from build123d import *

# Parameters (mm, degrees)
SKETCH1_W             = 45
SKETCH1_H             = 33
EXTRUDE1_DEPTH        = 45
EXTRUDE3_DEPTH        = 53.948087784
M5_TAPPED_HOLE1_D     = 4.2
M5_TAPPED_HOLE1_DEPTH = 10
M5_TAPPED_HOLE1_TIP   = 1.2618073
CHAMFER1_SIZE         = 1


with BuildPart() as part:
    # Sketch1 → Extrude1 (new body)
    with BuildSketch(Plane.XY):
        Rectangle(SKETCH1_W, SKETCH1_H)
    extrude(amount=EXTRUDE1_DEPTH)

    # Sketch2 → Extrude3 (cut, through all)
    with BuildSketch(Plane.XY.offset(45)):
        with BuildLine():
            Line((4.983173546, -10.386071552), (0, -4.447356576))
            Line((0, -4.447356576), (-4.983173546, -10.386071552))
            ThreePointArc((-4.983173546, -10.386071552), (0, -12), (4.983173546, -10.386071552))
        make_face()
        with BuildLine():
            Line((-4.983173546, -10.386071552), (0, -4.447356576))
            Line((0, -4.447356576), (4.983173546, -10.386071552))
            ThreePointArc((4.983173546, -10.386071552), (7.569906708, -7.366071964), (8.5, -3.5))
            ThreePointArc((8.5, -3.5), (-3.866071964, 4.069906708), (-4.983173546, -10.386071552))
        make_face()
        Polygon((10.113368652, -16.5), (-10.113368652, -16.5), (-13.53955506, -20.583169961), (13.53955506, -20.583169961), align=None)
        with BuildLine():
            ThreePointArc((4.983173546, -10.386071552), (0, -12), (-4.983173546, -10.386071552))
            Line((-4.983173546, -10.386071552), (-10.113368652, -16.5))
            Line((-10.113368652, -16.5), (10.113368652, -16.5))
            Line((10.113368652, -16.5), (4.983173546, -10.386071552))
        make_face()
    extrude(amount=-EXTRUDE3_DEPTH, mode=Mode.SUBTRACT)

    # M5 Tapped Hole1
    with Locations(Plane(origin=(0, 16.5, 0), x_dir=(-1, 0, 0), z_dir=(0, 1, 0))):
        with Locations((16, 7.5), (-16, 7.5), (-16, 37.5), (16, 37.5)):
            Hole(M5_TAPPED_HOLE1_D / 2, depth=M5_TAPPED_HOLE1_DEPTH)
            with Locations((0, 0, -(M5_TAPPED_HOLE1_DEPTH + M5_TAPPED_HOLE1_TIP / 2))):  # 118° drill point
                Cone(0, M5_TAPPED_HOLE1_D / 2, M5_TAPPED_HOLE1_TIP, mode=Mode.SUBTRACT)

    # Chamfer1
    chamfer1_edges = [part.edges().sort_by_distance(p)[0] for p in [
        (-22.5, 0, 45),
        (-16.306684326, -16.5, 45),
        (16.306684326, -16.5, 0),
        (16.306684326, -16.5, 45),
        (0, 5, 45),
        (0, 5, 0),
        (22.5, 0, 45),
        (-16.306684326, -16.5, 0),
        (-22.5, 0, 0),
        (0, 16.5, 0),
        (22.5, 0, 0),
        (0, 16.5, 45),
        (22.5, -16.5, 22.5),
        (-22.5, -16.5, 22.5),
        (-22.5, 16.5, 22.5),
        (22.5, 16.5, 22.5),
    ]]
    chamfer(chamfer1_edges, length=CHAMFER1_SIZE)


solid = part.part
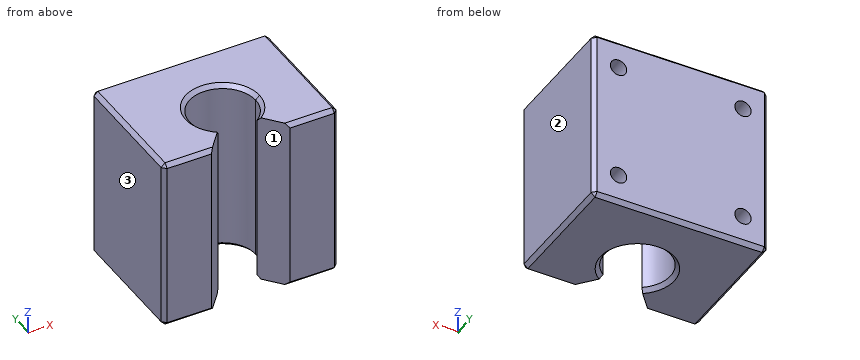
Model file for the job. Use its own axes, mm. Face numbers are marked on the shaded views. Give positions to 0.01 mm unless a question says otherwise; leave off trailing zeros. Order: outer loops, then holes, each group sorted by start corner. A loop starts at its lowest first (then second) coordinate and runs counter-clockwise, first axis right, second up. Notation, with made-up numbers: M 2.5,-39 L 18.5,-39 A11 ccw 18.5,-29 Z; hole C -20,42.25 d5. An arc over 180 degrees is marked long. Put each result on its own line as item: value. Start each with the question number.
(1) Band-saw the part on A-A on z = 17. Give the cut face in (x, y), then the cut area to 3 significant figures.
(2) Band-saw the part on B-B on x = 0. Give the cut face in (y, z), then the cut area to 4 significant figures.
(3) Drill centre lines: L1, parallel to Z at x = 16, y = 11; L2, parallel to X at y = 12.25, z = 7.5; L3, parallel to X at y = 15, z = 38. Where is each one in solid material? Low to high. Write a range as [from, to].
(4) Pull direction X, two halves, no side cores. Call the marked faces 1, 2 and 3: released by +X, released by -X, zero draft, split by the parting line, or undercut.
(5) Band-saw the part on C-C on y = -13.5. Give the cut face in (x, z).
(6) Pin check, flat tips, straight feed: pin 1 Ø4 at (x, z) = (16, 7.5) entering from +Y; pin 2 Ø5 at (x, z) = (5.5, 7.5) entering from -Y. Stop position of each tip, or through.
Results below:
1. outline: M -22.5,-15.5 L -21.5,-16.5 L -10.11,-16.5 L -4.98,-10.39 A8.5 cw long 4.98,-10.39 L 10.11,-16.5 L 21.5,-16.5 L 22.5,-15.5 L 22.5,15.5 L 21.5,16.5 L -21.5,16.5 L -22.5,15.5 Z
1. area: 1,170 mm2
2. outline: M 5,1 L 6,0 L 15.5,0 L 16.5,1 L 16.5,44 L 15.5,45 L 6,45 L 5,44 Z
2. area: 515.5 mm2
3. L1: z = [0, 5.4], [9.6, 35.4], [39.6, 45]
3. L2: x = [-22.5, -18.1], [-13.9, 13.9], [18.1, 22.5]
3. L3: x = [-22.5, -18.04], [-13.96, 13.96], [18.04, 22.5]
4. face 1: undercut
4. face 2: released by +X
4. face 3: released by -X
5. outline: M -22.5,1 L -21.5,0 L -7.6,0 L -7.6,45 L -21.5,45 L -22.5,44 Z; M 7.6,0 L 21.5,0 L 22.5,1 L 22.5,44 L 21.5,45 L 7.6,45 Z
6. pin 1: stops at y = 6.44
6. pin 2: stops at y = -13.98
